Build history of the part. All positions in model axes, mm. A direction names the side the tool comes from. Give positions to 0.01 mm unless a question says otherwise; leave off trailing zeros. Loops run counter-clockwise (first coordinate to the right, second up) from the corner with the lowest first, then second, coordinate; pieces in that order, holes last. Notation, with made-up numbers: M 44,49.25 L 69,49.25 A8 cw 69,62.25 Z; hole C 6,16.5 d6. An arc over 180 degrees is marked long. Answer in a Markdown table with one row per item. Add a question column.
```python
from build123d import *

# Parameters (mm, degrees)
BOSS_EXTRUDE1_DEPTH = 5
BOSS_EXTRUDE2_DEPTH = 3
SKETCH3_W           = 7.507408842
SKETCH3_H           = 20
BOSS_EXTRUDE3_DEPTH = 12
CUT_EXTRUDE2_DEPTH  = 18
SKETCH6_R           = 2
CUT_EXTRUDE3_DEPTH  = 48.063378728
SKETCH7_W           = 24.049396926
SKETCH7_H           = 4
CUT_EXTRUDE4_DEPTH  = 10
FILLET1_R           = 10


with BuildPart() as part:
    # Sketch1 → Boss-Extrude1 (new body)
    with BuildSketch(Plane(origin=(0, 0, 0), x_dir=(1, 0, 0), z_dir=(0, 1, 0))):
        Polygon((-10.454849344, 8.996116817), (-24.051323202, -14.553666709), (-16.16163723, -38.632828909), (16.16163723, -38.632828909), (24.051323202, -14.553666709), (10.454849344, 8.996116817), align=None)
        Polygon((9.300148806, 6.996116817), (-9.300148806, 6.996116817), (-21.872561183, -14.779940194), (-14.712327446, -36.632828909), (14.712327446, -36.632828909), (21.872561183, -14.779940194), align=None, mode=Mode.SUBTRACT)
    extrude(amount=BOSS_EXTRUDE1_DEPTH)

    # Sketch2 → Boss-Extrude2 (add)
    with BuildSketch(Plane(origin=(0, 0, 0), x_dir=(-1, 0, 0), z_dir=(0, -1, 0))):
        Polygon((24.051323202, -14.553666709), (10.454849344, 8.996116817), (-10.454849344, 8.996116817), (-24.051323202, -14.553666709), (-16.16163723, -38.632828909), (16.16163723, -38.632828909), align=None)
    extrude(amount=BOSS_EXTRUDE2_DEPTH)

    # Sketch3 → Boss-Extrude3 (add)
    with BuildSketch(Plane(origin=(0, -3, 0), x_dir=(-1, 0, 0), z_dir=(0, -1, 0))):
        with Locations((9.003704421, -17.503883183)):
            Rectangle(SKETCH3_W, SKETCH3_H)
        with Locations((-9.003704421, -17.503883183)):
            Rectangle(SKETCH3_W, SKETCH3_H)
    extrude(amount=BOSS_EXTRUDE3_DEPTH)

    # Sketch5 → Cut-Extrude2 (cut)
    with BuildSketch(Plane(origin=(0, 0, 7.503883183), x_dir=(-1, 0, 0), z_dir=(0, 0, -1))):
        Polygon((-9.75, -13), (9.75, -13), (9.75, -10.85), (6.75, -10.85), (6.75, -3), (5.25, -3), (5.25, -10.85), (-5.25, -10.85), (-5.25, -3), (-6.75, -3), (-6.75, -10.85), (-9.75, -10.85), align=None)
    extrude(amount=-CUT_EXTRUDE2_DEPTH, mode=Mode.SUBTRACT)

    # Sketch6 → Cut-Extrude3 (cut, through all)
    with BuildSketch(Plane(origin=(0, -3, 0), x_dir=(-1, 0, 0), z_dir=(0, -1, 0))):
        with Locations(Location((-15.327870678, -13.003883183, 0), (0, 0, 90))):
            Circle(SKETCH6_R)
        with Locations(Location((15.327870678, -13.003883183, 0), (0, 0, 90))):
            Circle(SKETCH6_R)
        Polygon((-5.25, -38.632828909), (5.25, -38.632828909), (5.25, -25.503883183), (6.75, -25.503883183), (6.75, -4.503883183), (-6.75, -4.503883183), (-6.75, -25.503883183), (-5.25, -25.503883183), align=None)
    extrude(amount=-CUT_EXTRUDE3_DEPTH, mode=Mode.SUBTRACT)

    # Sketch7 → Cut-Extrude4 (cut)
    with BuildSketch(Plane(origin=(0, -3, 0), x_dir=(-1, 0, 0), z_dir=(0, -1, 0))):
        with Locations((0, 8.496116817)):
            Rectangle(SKETCH7_W, SKETCH7_H)
    extrude(amount=-CUT_EXTRUDE4_DEPTH, mode=Mode.SUBTRACT)

    # Fillet1
    fillet1_edges = [part.edges().sort_by_distance(p)[0] for p in [
        (-11.898225017, 1, -6.496116817),
        (11.898225017, 1, -6.496116817),
    ]]
    fillet(fillet1_edges, radius=FILLET1_R)


solid = part.part
```
(1) Slice it at D-D, the plane y = 0.75. Give the cut face in (x, z).
(2) Wall check: line 1 (X direction, y = -9, z = 22.5); line 2 (Y direction, x = 7.5, z = 10.5); line 3 (Z direction, x = -3, y = -1). Give the ranges that are in metal, low to high.
(3) Pin check, flat tips, straight feed: pin 1 (10 mm diameter, centred on y = -10, z = 17.5, fed in from -X); pin 2 (10 mm diameter, centred on y = 0, z = 21, fed in from +X); pin 3 (6 mm diameter, centred on y = -4.5, z = 32.5, fed in from -X); pin 4 (9.5 mm diameter, centred on y = -7.5, z = 14, fed in from +X). Stop position of each tip, or through.
(4) Tool access for faces 1 (the flat face through (-18.343, 2.465, 25.553)), 2 (the flat face through (-12.757, -9, 18)), 3 (the flat face through (10, -9, 7.504)): list every direction of +Z, -Z, +X, -X, +Y, -Y with a clear straight run to the whole face (end or side of a thin tool).
(5) Pull direction X, two halves, no side cores. Call faces 4 (the flat face through (19.353, 1.056, 6.416)), 5 (the flat face through (-20.05, 1.06, 26.76)), 6 (the flat face through (-9, -15, 17)), 7 (the flat face through (-8, -10.85, 16)): +X half, -X half, draft (parallel to the pull), parting line (faces both ways), or undercut.
(6) Slice it at B-B, the plane z = 14. State how many separate pieces and enclosed holes the cut face has, then the cut area to 3 significant figures.
(7) Slice it at A-A, the plane y = -6. Give the cut face in (x, z).
(8) Slice it at C-C, the plane z = 30. Give the cut face in (x, y).
Solution:
| question | item | result |
|---|---|---|
| 1 | outline | M -24.05,14.55 L -14.78,-1.5 A10 ccw -10.05,-5.69 L -21.87,14.78 L -14.71,36.63 L -5.25,36.63 L -5.25,38.63 L -16.16,38.63 Z; M 5.25,36.63 L 14.71,36.63 L 21.87,14.78 L 10.05,-5.69 A10 ccw 14.78,-1.5 L 24.05,14.55 L 16.16,38.63 L 5.25,38.63 Z |
| 2 | line 1 | -12.76 to -6.75, 6.75 to 12.76 |
| 2 | line 2 | -15 to -13, -10.85 to 0 |
| 2 | line 3 | -6.5 to 4.5 |
| 3 | pin 1 | x = -12.76 |
| 3 | pin 2 | x = 23.58 |
| 3 | pin 3 | x = -19.02 |
| 3 | pin 4 | x = 24.05 |
| 4 | face 1 | +Y |
| 4 | face 2 | +Z, -Z, -X, -Y |
| 4 | face 3 | -Z, +X, -X, -Y |
| 5 | face 4 | +X half |
| 5 | face 5 | -X half |
| 5 | face 6 | draft |
| 5 | face 7 | undercut |
| 6 | separate pieces | 4 |
| 6 | enclosed holes | 0 |
| 6 | area | 241 mm^2 |
| 7 | outline | M -12.76,7.5 L -6.75,7.5 L -6.75,25.5 L -5.25,25.5 L -5.25,27.5 L -12.76,27.5 Z; M 5.25,25.5 L 6.75,25.5 L 6.75,7.5 L 12.76,7.5 L 12.76,27.5 L 5.25,27.5 Z |
| 8 | outline | M -18.99,-3 L -5.25,-3 L -5.25,0 L -16.89,0 L -16.89,5 L -18.99,5 Z; M 5.25,-3 L 18.99,-3 L 18.99,5 L 16.89,5 L 16.89,0 L 5.25,0 Z |
